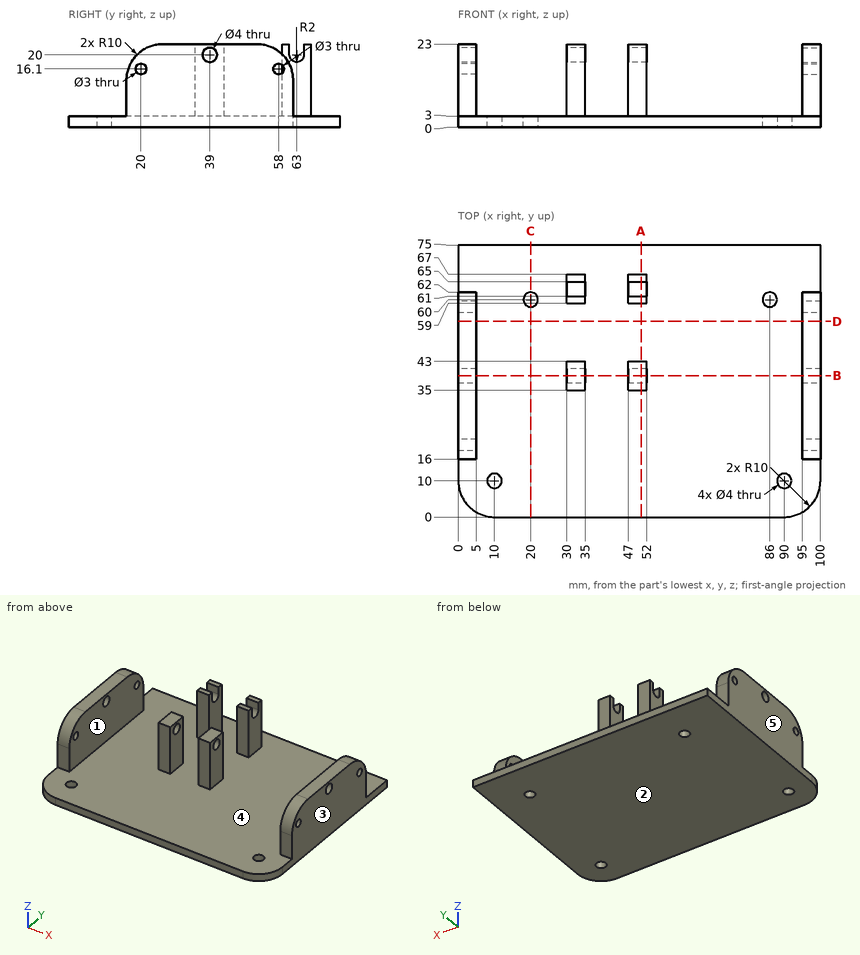
Answer from the drawing. Dimensions are ordinates in mm from the lowest x, y and z of the part. A direction names the side the tool comes from. Round coordinates to 2 decimals unless told otherwise and drop trailing zeros. Loops run counter-clockwise (first coordinate to the right, second up) from the corner with the lowest first, then second, coordinate; pieces in that order, holes last.
Q1. Which of the six approach directions +Z, -Z, +X, -X, +Y, -Y give full straight-line access (tool end or side, diameter ignored) to the marked faces 1 and 2?
Q2. Section D-D on y = 54 is taken. Write down the section's boundary in (x, z), and give its area (3 significant figures).
Q3. Section A-A on x = 50.5 is taken. Write down the section's boundary in (y, z).
Q4. Section C-C on x = 20 is taken. Write down the section's boundary in (y, z), and give its area (3 significant figures).
Q5. Each of these flat-tipped pins is pushed along its axis until it touches: pin 1 (3.5 mm diameter, centred on x = 32, z = 22, fed in from +Y); pin 2 (4.5 mm diameter, centred on x = 20, y = 60, fed in from +Z); pin 3 (1.5 mm diameter, centred on x = 49, z = 8, fed in from -Y). Where does it stop, or does it pass through?
Q6. Consider probe 1 along X at (y, z) = (29, 16); probe 2 along Z at (x, y) = (2.5, 39); probe 3 along X at (y, z) = (64, 16.25). Determine where each line is inside the solid, lowest interval first.
Q7. Determine the mould class of the marked faces 3, 4 and 5 for opening direction X: released by +X, released by -X, zero draft, split by the parting line, or undercut.
Q8. Section B-B on y = 39 is taken. Give the number of separate pieces and of enclosed holes in the cut face, and give its area (3 significant figures).
Output:
1. face 1: +Z, +Y, -Y
1. face 2: -Z, +X, -X, +Y, -Y
2. outline: (0, 0) - (100, 0) - (100, 22.8) - (95, 22.8) - (95, 3) - (5, 3) - (5, 22.8) - (0, 22.8) - close
2. area: 498 mm2
3. outline: (0, 0) - (75, 0) - (75, 3) - (67, 3) - (67, 23) - (65, 23) - (65, 20) arc R2 cw to (61, 20) - (61, 23) - (59, 23) - (59, 3) - (43, 3) - (43, 23) - (35, 23) - (35, 3) - (0, 3) - close; hole circle Ø4 at (39, 20)
4. outline: (0, 0) - (58, 0) - (58, 3) - (0, 3) - close; (62, 0) - (75, 0) - (75, 3) - (62, 3) - close
4. area: 213 mm2
5. pin 1: stops at y = 67
5. pin 2: stops at z = 3
5. pin 3: stops at y = 35
6. probe 1: x = 0 to 5, 95 to 100
6. probe 2: z = 0 to 18, 22 to 23
6. probe 3: x = 30 to 35, 47 to 52
7. face 3: released by +X
7. face 4: undercut
7. face 5: released by -X
8. separate pieces: 5
8. enclosed holes: 0
8. area: 620 mm2
